The listing builds one solid part. Answer for the finished solid, in the listing's coordinates (mm). Give positions to 0.01 mm unless a question says otherwise; leave off trailing zeros. Answer as CSV lines item,"result". Start each with the question number.
(1) Each of these flat-tipped pins is pushed along its axis until it touches: pin 1 Ø6 at (x, z) = (-10, -93) entering from +Y; pin 2 Ø5 at (x, y) = (-4.5, 2.5) entering from -Z; pin 3 Ø0.8 at (x, z) = (-14, -60.5) entering from +Y; pin 4 Ø6 at (x, z) = (-11.5, 132.5) entering from -Y. Where does it stop, or does it pass through?
(2) Find section A-A (z = 128.5). State how many separate pieces and enclosed holes the cut face has, then the cut area to 3 significant figures.
(3) For a pull along Z with two mould halves and no side action, classify faces 1 (the face through (0, -10, 4)), 2 (the face through (4.4, -5.1, 250)), 3 (the face through (4.4, -5.1, -250)) as pulls with the +Z half, pulls with the -Z half, needs draft (parallel to the pull), parting line crosses it, or undercut.
(4) Straight lines are drawn through the part: probe 1 along Y at (x, z) = (18, -27); probe 2 along Y at (x, z) = (5, 26); probe 3 along X at (y, z) = (-6.5, -152.5). For each, find the intervals that lie inside material, in ascending order.
Autodesk Inventor part; units mm, degrees
ref_plane "Work Plane2" through (-5.36, -10, 250) normal (0, 0, 1) x (1, 0, 0)
ref_plane "YZ Plane" through (0, 0, 0) normal (1, 0, 0) x (0, 1, 0)
ref_plane "XZ Plane" through (0, 0, 0) normal (0, 1, 0) x (-1, 0, 0)
ref_plane "Work Plane2" through (-5.36, -10, 250) normal (0, 0, 1) x (1, 0, 0)
sketch "Sketch1" plane through (-5.36, -10, 250) normal (0, 0, 1) x (1, 0, 0)
  line L0 (-1.8, 13.9007) -> (-7.48, 13.9007)
  line L1 (-7.48, 13.9007) -> (-10.1393, 16.56)
  line L2 (-10.1393, 16.56) -> (-10.1393, 18.2)
  line L3 (-10.1393, 18.2) -> (-7.48, 18.2)
  line L4 (-7.48, 18.2) -> (-9.28, 20)
  line L5 (-9.28, 20) -> (-12.84, 20)
  arc A0 (-12.84, 20) -> (-14.64, 18.2) centre (-12.84, 18.2) ccw
  line L6 (-14.64, 18.2) -> (-14.64, 14.64)
  line L7 (-14.64, 14.64) -> (-12.84, 12.84)
  line L8 (-12.84, 12.84) -> (-12.84, 15.4993)
  line L9 (-12.84, 15.4993) -> (-11.2, 15.4993)
  line L10 (-11.2, 15.4993) -> (-8.5407, 12.84)
  line L11 (-8.5407, 12.84) -> (-8.5407, 7.16)
  line L12 (-8.5407, 7.16) -> (-11.2, 4.5007)
  line L13 (-11.2, 4.5007) -> (-12.84, 4.5007)
  line L14 (-12.84, 4.5007) -> (-12.84, 7.16)
  line L15 (-12.84, 7.16) -> (-14.64, 5.36)
  line L16 (-14.64, 5.36) -> (-14.64, 1.8)
  arc A1 (-14.64, 1.8) -> (-12.84, 0) centre (-12.84, 1.8) ccw
  line L17 (-12.84, 0) -> (-9.28, 0)
  line L18 (-9.28, 0) -> (-7.48, 1.8)
  line L19 (-7.48, 1.8) -> (-10.1393, 1.8)
  line L20 (-10.1393, 1.8) -> (-10.1393, 3.44)
  line L21 (-10.1393, 3.44) -> (-7.48, 6.0993)
  line L22 (-7.48, 6.0993) -> (-1.8, 6.0993)
  line L23 (-1.8, 6.0993) -> (0.8593, 3.44)
  line L24 (0.8593, 3.44) -> (0.8593, 1.8)
  line L25 (0.8593, 1.8) -> (-1.8, 1.8)
  line L26 (-1.8, 1.8) -> (0, 0)
  line L27 (0, 0) -> (10.72, 0)
  line L28 (10.72, 0) -> (12.52, 1.8)
  line L29 (12.52, 1.8) -> (9.8607, 1.8)
  line L30 (9.8607, 1.8) -> (9.8607, 3.44)
  line L31 (9.8607, 3.44) -> (12.52, 6.0993)
  line L32 (12.52, 6.0993) -> (18.2, 6.0993)
  line L33 (18.2, 6.0993) -> (20.8593, 3.44)
  line L34 (20.8593, 3.44) -> (20.8593, 1.8)
  line L35 (20.8593, 1.8) -> (18.2, 1.8)
  line L36 (18.2, 1.8) -> (20, 0)
  line L37 (20, 0) -> (23.56, 0)
  arc A2 (23.56, 0) -> (25.36, 1.8) centre (23.56, 1.8) ccw
  line L38 (25.36, 1.8) -> (25.36, 5.36)
  line L39 (25.36, 5.36) -> (23.56, 7.16)
  line L40 (23.56, 7.16) -> (23.56, 4.5007)
  line L41 (23.56, 4.5007) -> (21.92, 4.5007)
  line L42 (21.92, 4.5007) -> (19.2607, 7.16)
  line L43 (19.2607, 7.16) -> (19.2607, 12.84)
  line L44 (19.2607, 12.84) -> (21.92, 15.4993)
  line L45 (21.92, 15.4993) -> (23.56, 15.4993)
  line L46 (23.56, 15.4993) -> (23.56, 12.84)
  line L47 (23.56, 12.84) -> (25.36, 14.64)
  line L48 (25.36, 14.64) -> (25.36, 18.2)
  arc A3 (25.36, 18.2) -> (23.56, 20) centre (23.56, 18.2) ccw
  line L49 (23.56, 20) -> (20, 20)
  line L50 (20, 20) -> (18.2, 18.2)
  line L51 (18.2, 18.2) -> (20.8593, 18.2)
  line L52 (20.8593, 18.2) -> (20.8593, 16.56)
  line L53 (20.8593, 16.56) -> (18.2, 13.9007)
  line L54 (18.2, 13.9007) -> (12.52, 13.9007)
  line L55 (12.52, 13.9007) -> (9.8607, 16.56)
  line L56 (9.8607, 16.56) -> (9.8607, 18.2)
  line L57 (9.8607, 18.2) -> (12.52, 18.2)
  line L58 (12.52, 18.2) -> (10.72, 20)
  line L59 (10.72, 20) -> (0, 20)
  line L60 (0, 20) -> (-1.8, 18.2)
  line L61 (-1.8, 18.2) -> (0.8593, 18.2)
  line L62 (0.8593, 18.2) -> (0.8593, 16.56)
  line L63 (0.8593, 16.56) -> (-1.8, 13.9007)
  circle A4 centre (-4.64, 10) radius 2.1
  line L64 (-12.84, 1.8) -> (-11.2093, 1.8)
  line L65 (-12.84, 3.4307) -> (-12.84, 1.8)
  line L66 (-12.27, 3.4307) -> (-12.84, 3.4307)
  line L67 (-11.2093, 2.37) -> (-12.27, 3.4307)
  line L68 (-11.2093, 1.8) -> (-11.2093, 2.37)
  line L69 (23.56, 16.5693) -> (23.56, 18.2)
  line L70 (22.99, 16.5693) -> (23.56, 16.5693)
  line L71 (21.9293, 17.63) -> (22.99, 16.5693)
  line L72 (21.9293, 18.2) -> (21.9293, 17.63)
  line L73 (23.56, 18.2) -> (21.9293, 18.2)
  circle A5 centre (15.36, 10) radius 2.1
  line L74 (23.56, 1.8) -> (23.56, 3.4307)
  line L75 (21.9293, 1.8) -> (23.56, 1.8)
  line L76 (21.9293, 2.37) -> (21.9293, 1.8)
  line L77 (22.99, 3.4307) -> (21.9293, 2.37)
  line L78 (23.56, 3.4307) -> (22.99, 3.4307)
  line L79 (-11.2093, 18.2) -> (-12.84, 18.2)
  line L80 (-11.2093, 17.63) -> (-11.2093, 18.2)
  line L81 (-12.27, 16.5693) -> (-11.2093, 17.63)
  line L82 (-12.84, 16.5693) -> (-12.27, 16.5693)
  line L83 (-12.84, 18.2) -> (-12.84, 16.5693)
  line L84 (8.06, 18.2) -> (2.66, 18.2)
  line L85 (8.06, 16.2393) -> (8.06, 18.2)
  line L86 (11.4593, 12.84) -> (8.06, 16.2393)
  line L87 (11.4593, 7.16) -> (11.4593, 12.84)
  line L88 (8.06, 3.7607) -> (11.4593, 7.16)
  line L89 (8.06, 1.8) -> (8.06, 3.7607)
  line L90 (2.66, 1.8) -> (8.06, 1.8)
  line L91 (2.66, 3.7607) -> (2.66, 1.8)
  line L92 (-0.7393, 7.16) -> (2.66, 3.7607)
  line L93 (-0.7393, 12.84) -> (-0.7393, 7.16)
  line L94 (2.66, 16.2393) -> (-0.7393, 12.84)
  line L95 (2.66, 18.2) -> (2.66, 16.2393)
  point P0 (5.36, 10)
extrude "Extrusion2" add sketch "Sketch1" against normal blind 500
properties part number "vslot_20x40x500"
Result set:
1,pin 1,"y = 8.36"
1,pin 2,"z = -250"
1,pin 3,"y = 9.76"
1,pin 4,"y = -9.86"
2,separate pieces,"1"
2,enclosed holes,"7"
2,area,"289 mm^2"
3,face 1,"needs draft"
3,face 2,"pulls with the +Z half"
3,face 3,"pulls with the -Z half"
4,probe 1,"-10 to -8.2, -6.57 to -5.5, 5.5 to 6.57, 8.2 to 10"
4,probe 2,"-10 to -8.2, -6.06 to -3.94, 3.94 to 6.06, 8.2 to 10"
4,probe 3,"-20 to -15.44, -4.56 to -2.7, 2.7 to 4.56, 15.44 to 20"
